Build history of the part. All positions in model axes, mm. A direction names the side the tool comes from. Coordinates: 2 decimals unless noted, no trailing zeros. Write each loop counter-clockwise with the first axis right and the second up, starting at its lowest first coordinate (ties: lowest second). Pieces come first, ordered by that corner, then holes.
```python
from build123d import *

# Parameters (mm, degrees)
F0_R     = 16.5
F1_DEPTH = 22
F0_R_2   = 37.5
F2_DEPTH = 26
F3_DEPTH = 4


# Not quite as in the source:
# - a feature names something its author has since deleted; it is built from what else it names


with BuildPart() as f1:
    # F0 (on Top) → F1 (new body)
    with BuildSketch(Plane.XY):
        Circle(F0_R)
        Polygon((3.7527767497, 0), (1.8763883749, -3.25), (-1.8763883749, -3.25), (-3.7527767497, 0), (-1.8763883749, 3.25), (1.8763883749, 3.25), align=None, mode=Mode.SUBTRACT)
    extrude(amount=F1_DEPTH)

    # F0 (on Top) → F2 (join)
    with BuildSketch(Plane.XY):
        Circle(F0_R_2)
        Circle(F0_R, mode=Mode.SUBTRACT)
    extrude(amount=F2_DEPTH)

    # F0 (on Top) → F3 (join)
    with BuildSketch(Plane.XY):
        Circle(F0_R_2)
        Circle(F0_R, mode=Mode.SUBTRACT)
    extrude(amount=-F3_DEPTH)


solid = f1.part
```
1. Mould opens along Y. For faces 1 (the face through (-4.88, 37.18, 11.21)), 2 (the face through (8, -16, 26)), 3 (the face through (-2.8, -1.65, 10.85)) say: +Y half, -Y half, draft (parallel to the pull), parting line (faces both ways), or undercut.
Computed values:
face 1: parting line
face 2: draft
face 3: undercut
2. Probe line 1 along Y through (x, z) = (0, 23.65); line 2 along Z through (x, y) = (-8.5, -12.5); line 3 along X through (y, z) = (11, 22.5). List the from-to ranges inside material, lowest first.
Computed values:
line 1: y = -37.5 to -16.5, 16.5 to 37.5
line 2: z = 0 to 22
line 3: x = -35.85 to -12.3, 12.3 to 35.85
3. Saw through at A-A on x = 0. List the corners of the cut face in (y, z).
Computed values:
outline: (-37.5, -4) - (-16.5, -4) - (-16.5, 0) - (-3.25, 0) - (-3.25, 22) - (-16.5, 22) - (-16.5, 26) - (-37.5, 26) - close; (3.25, 0) - (16.5, 0) - (16.5, -4) - (37.5, -4) - (37.5, 26) - (16.5, 26) - (16.5, 22) - (3.25, 22) - close
4. Saw through at C-C on y = -12. List the corners of the cut face in (x, z).
Computed values:
outline: (-35.53, -4) - (-11.32, -4) - (-11.32, 0) - (11.32, 0) - (11.32, -4) - (35.53, -4) - (35.53, 26) - (11.32, 26) - (11.32, 22) - (-11.32, 22) - (-11.32, 26) - (-35.53, 26) - close
5. Saw through at B-B on z = 17. List the corners of the cut face in (x, y).
Computed values:
outline: circle Ø75 at (0, 0); hole (-3.75, 0) - (-1.88, -3.25) - (1.88, -3.25) - (3.75, 0) - (1.88, 3.25) - (-1.88, 3.25) - close
6. Flat gauge pins, fed straight in: pin 1 (8 mm diameter, centred on y = -26.5, z = 11, fed in from -X); pin 2 (6 mm diameter, centred on y = -7.5, z = 22.5, fed in from +X); pin 3 (3 mm diameter, centred on x = -7.5, z = 17.5, fed in from -Y). Where does each tip first touch, or does it go through?
Computed values:
pin 1: stops at x = -30
pin 2: stops at x = 37.23
pin 3: stops at y = -37.02
7. 3-axis set-ups, long thin cutter, end or side, ignore diameter. For faces 4 (the face through (2.8, 1.65, 10.85)), 5 (the face through (-0.23, -3.44, 0)), 6 (the face through (8, -16, -4)), 7 (the face through (-0.23, -3.44, 22)): which of +Z, -Z, +X, -X, +Y, -Y reach the whole face in a straight line?
Computed values:
face 4: +Z, -Z
face 5: -Z
face 6: -Z, +X, -X, +Y, -Y
face 7: +Z
8. Saw through at D-D on x = -8. List the corners of the cut face in (y, z), plus the area to 3 significant figures.
Computed values:
outline: (-36.64, -4) - (-14.43, -4) - (-14.43, 0) - (14.43, 0) - (14.43, -4) - (36.64, -4) - (36.64, 26) - (14.43, 26) - (14.43, 22) - (-14.43, 22) - (-14.43, 26) - (-36.64, 26) - close
area: 1,970 mm2
